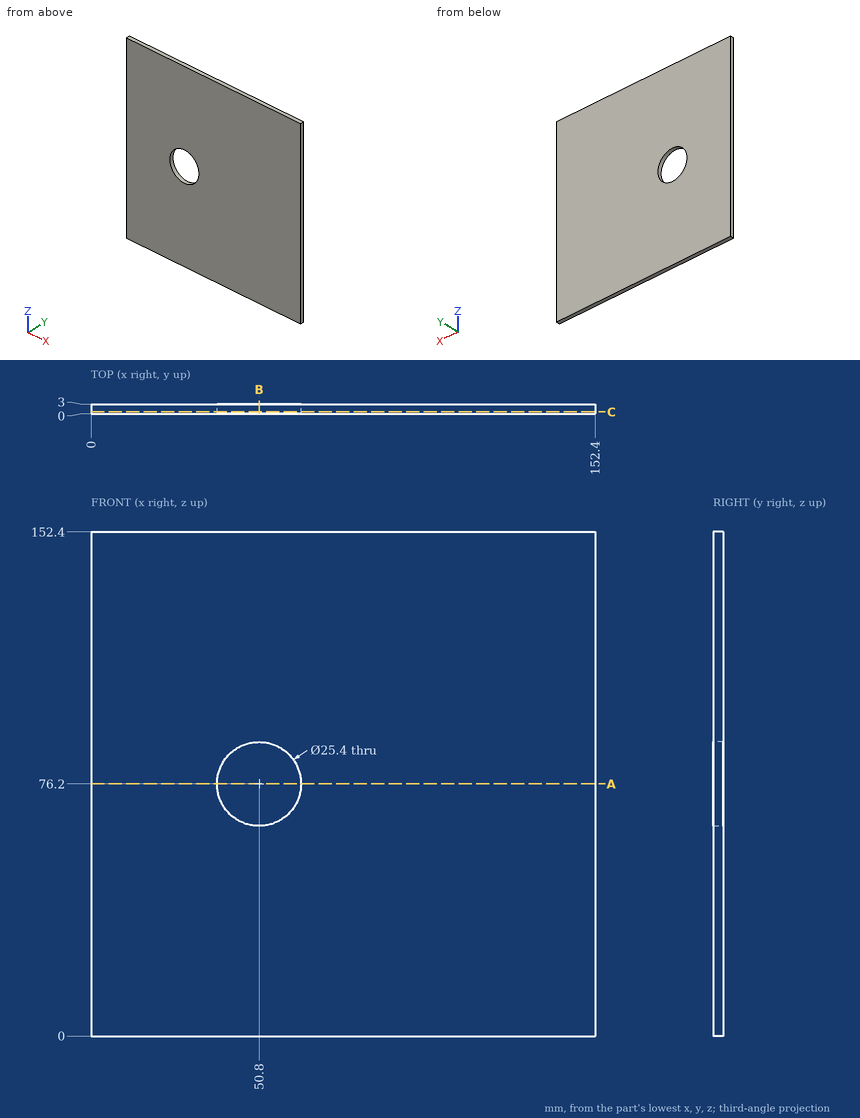
Could you check a few things on this drawing? It's one solid part, dimensions in mm from its lowest x, y, z. Coordinates: 2 decimals unless noted, no trailing zeros. Loops run counter-clockwise (first coordinate to the right, second up) from the corner with the lowest first, then second, coordinate; pieces in that order, holes last. Notation, with made-up numbers: (68, 64) - (116, 64) arc R4 ccw to (116, 71) - close; hole circle Ø9 at (-27, 55.5). An arc over 180 degrees is marked (long way). Return JSON: item names as keys, results as strings. Group by question number.
Item 1: Will this pin go through, and if not, where does the flat tip stop? P1, Ø23, axis at x = 50.8, z = 76.2, coming from the -Y side.
Item 2: I need wall thicknesses on line 1 (X direction, y = 2, z = 76.2); line 2 (X direction, y = 1.85, z = 69.5); line 3 (Z direction, x = 52.5, y = 1). Which ranges of each line are inside material? Lowest first, please. Write a range as from..to.
Item 3: If we section it at A-A on z = 76.2: Write out the boundary of the cut face in (x, y).
Item 4: If we section it at C-C on y = 0.65: Write out the boundary of the cut face in (x, z), and give its area (3 significant figures).
Item 5: If we section it at B-B on x = 50.8: Write out the boundary of the cut face in (y, z), and give its area (3 significant figures).
Calculated:
{
 "1": {"P1": "passes through"},
 "2": {"line 1": "x = 0..38.1, 63.5..152.4", "line 2": "x = 0..40.01, 61.59..152.4", "line 3": "z = 0..63.61, 88.79..152.4"},
 "3": {"outline": "(0, 0) - (38.1, 0) - (38.1, 3) - (0, 3) - close; (63.5, 0) - (152.4, 0) - (152.4, 3) - (63.5, 3) - close"},
 "4": {"outline": "(0, 0) - (152.4, 0) - (152.4, 152.4) - (0, 152.4) - close; hole circle Ø25.4 at (50.8, 76.2)", "area": "22,700 mm^2"},
 "5": {"outline": "(0, 0) - (3, 0) - (3, 63.5) - (0, 63.5) - close; (0, 88.9) - (3, 88.9) - (3, 152.4) - (0, 152.4) - close", "area": "381 mm^2"}
}
